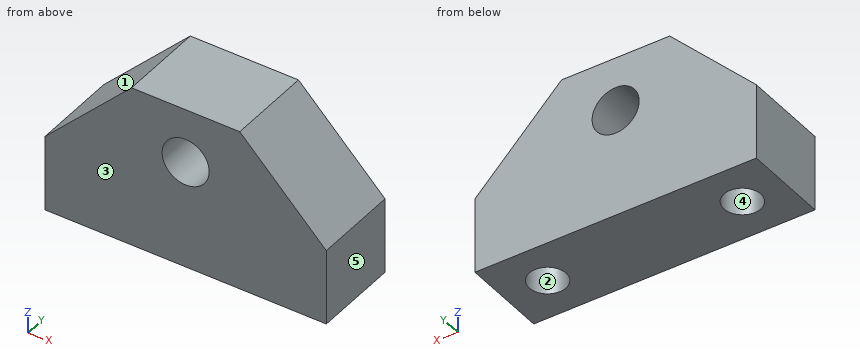
```python
from build123d import *

# Parameters (mm, degrees)
F0_W     = 20.6375
F0_H     = 6.35
F0_R     = 1.35255
F1_DEPTH = 4.7625
F2_W     = 20.6375
F2_H     = 6.35
F3_DEPTH = 7.14375
F4_SIZE  = 6.35
F5_R     = 1.7272
F6_DEPTH = 6.35


with BuildPart() as f1:
    # F0 (on Top) → F1 (new body)
    with BuildSketch(Plane.XY):
        with Locations((10.31875, 3.175)):
            Rectangle(F0_W, F0_H)
        with Locations((3.175, 3.175)):
            Circle(F0_R, mode=Mode.SUBTRACT)
        with Locations((17.4625, 3.175)):
            Circle(F0_R, mode=Mode.SUBTRACT)
    extrude(amount=F1_DEPTH)

    # F2 (on face) → F3 (join)
    with BuildSketch(Plane.XY.offset(4.7625)):
        with Locations((10.31875, 3.175)):
            Rectangle(F2_W, F2_H)
    extrude(amount=F3_DEPTH)

    # F4
    f4_edges = [f1.edges().sort_by_distance(p)[0] for p in [
        (20.6375, 3.175, 11.90625),
        (0, 3.175, 11.90625),
    ]]
    chamfer(f4_edges, length=F4_SIZE)

    # F5 (on face) → F6 (cut, through all)
    with BuildSketch(Plane(origin=(0, 6.35, 0), x_dir=(-1, 0, 0), z_dir=(0, 1, 0))):
        with Locations((-10.31875, 7.9375)):
            Circle(F5_R)
    extrude(amount=-F6_DEPTH, mode=Mode.SUBTRACT)


solid = f1.part
```
Geometry: final body of the model. Coordinates: model frame, mm. Face numbers are marked on the shaded views. A direction names the side the tool comes from. Round coordinates to 2 decimals unless told otherwise and drop trailing zeros. Loops run counter-clockwise (first coordinate to the right, second up) from the corner with the lowest first, then second, coordinate; pieces in that order, holes last. Notation, with made-up numbers: (-38, -39) -> (-3, -39) arc R8 cw to (-3, -28) -> close; hole circle Ø1 at (77.5, 50). An arc over 180 degrees is marked (long way). Write each question's results on one line, items separated by ' | '.
Item 1: Cut plane B-B on y = 0.5. Return the cut outline in (x, z), and give its area (3 significant figures).
Answers below:
outline: (0, 0) -> (20.64, 0) -> (20.64, 5.56) -> (14.29, 11.91) -> (6.35, 11.91) -> (0, 5.56) -> close; hole circle Ø3.45 at (10.32, 7.94) | area: 196 mm²
Item 2: Pin query (flat end, axial travel): pin 1 Ø3.5 at (x, y) = (3.175, 3.175) entering from +Z; pin 2 Ø3 at (x, z) = (10.32, 7.94) entering from +Y. Return the tip coordinate at first contact, or that it passes through.
Answers below:
pin 1: stops at z = 10.48 | pin 2: passes through
Item 3: Cut plane A-A on z = 9.25. Return the cut outline in (x, y), and give its area (3 significant figures).
Answers below:
outline: (3.69, 0) -> (9.2, 0) -> (9.2, 6.35) -> (3.69, 6.35) -> close; (11.44, 0) -> (16.94, 0) -> (16.94, 6.35) -> (11.44, 6.35) -> close | area: 69.9 mm²
Item 4: Cut plane C-C on x = 9. Return the cut outline in (y, z), and give its area (3 significant figures).
Answers below:
outline: (0, 0) -> (6.35, 0) -> (6.35, 6.82) -> (0, 6.82) -> close; (0, 9.05) -> (6.35, 9.05) -> (6.35, 11.91) -> (0, 11.91) -> close | area: 61.4 mm²
Item 5: Pull-direction query (X, two-part tool) for the marked faces 1, 2 and 3; classes: pulls with the +X half, pulls with the -X half, needs draft (parallel to the pull), parting line crosses it, or undercut.
Answers below:
face 1: pulls with the -X half | face 2: undercut | face 3: needs draft
Item 6: Set-up query: the marked faces 4 and 5. Return all of +Z, -Z, +X, -X, +Y, -Y with unobstructed straight access to the full face (end or side cutting, diameter ignored); none if empty.
Answers below:
face 4: -Z | face 5: +Z, -Z, +X, +Y, -Y
Item 7: Cut plane D-D on x = 18. Return the cut outline in (y, z), and give its area (3 significant figures).
Answers below:
outline: (0, 0) -> (1.93, 0) -> (1.93, 4.76) -> (4.42, 4.76) -> (4.42, 0) -> (6.35, 0) -> (6.35, 8.19) -> (0, 8.19) -> close | area: 40.2 mm²
Item 8: Line query: probe 1 along Y at (x, z) = (3.25, 0.75); probe 2 along X at (y, z) = (1.5, 8.25); probe 3 along Y at (x, z) = (4.25, 2). Output: solid intervals per line, ascending. Write a range as [from, to].
Answers below:
probe 1: y = [0, 1.82], [4.53, 6.35] | probe 2: x = [2.69, 8.62], [12.02, 17.94] | probe 3: y = [0, 2.35], [4, 6.35]
